from build123d import *

# Parameters (mm, degrees)
F1_DEPTH  = 15.875
F2_R      = 38.1
F3_DEPTH  = 31.751
F5_DEPTH  = 25.4
F6_R      = 12.7
F7_DEPTH  = 152.401
F9_DEPTH  = 25.4
F10_R     = 12.7
F11_DEPTH = 152.401
F14_DEPTH = 152.401


with BuildPart() as f1:
    # F0 (on Front) → F1 (new body, symmetric)
    with BuildSketch(Plane.XZ):
        with BuildLine():
            Line((88.9, 76.2), (0, 76.2))
            ThreePointArc((0, 76.2), (-76.2, 0), (0, -76.2))
            Line((0, -76.2), (88.9, -76.2))
            Line((88.9, -76.2), (88.9, 76.2))
        make_face()
    extrude(amount=F1_DEPTH, both=True)

    # F2 (on face) → F3 (cut, through all)
    with BuildSketch(Plane.XZ.offset(15.875)):
        Circle(F2_R)
    extrude(amount=-F3_DEPTH, mode=Mode.SUBTRACT)

    # F4 (on face) → F5 (join)
    with BuildSketch(Plane.XY.offset(76.2)):
        with BuildLine():
            ThreePointArc((114.3, -15.875), (142.540126, -23.966517), (159.527869, 0))
            ThreePointArc((159.527869, 0), (142.540126, 23.966517), (114.3, 15.875))
            ThreePointArc((114.3, 15.875), (108.727869, 0), (114.3, -15.875))
        make_face()
        with BuildLine():
            Line((114.3, 15.875), (88.9, 15.875))
            Line((88.9, 15.875), (88.9, -15.875))
            Line((88.9, -15.875), (114.3, -15.875))
            ThreePointArc((114.3, -15.875), (108.727869, 0), (114.3, 15.875))
        make_face()
    extrude(amount=-F5_DEPTH)

    # F6 (on face) → F7 (cut, through all)
    with BuildSketch(Plane(origin=(0, 0, -76.2), x_dir=(1, 0, 0), z_dir=(0, 0, -1))):
        with Locations((134.127869, 0)):
            Circle(F6_R)
    extrude(amount=-F7_DEPTH, mode=Mode.SUBTRACT)

    # F8 (on face) → F9 (join)
    with BuildSketch(Plane(origin=(0, 0, -76.2), x_dir=(1, 0, 0), z_dir=(0, 0, -1))):
        with BuildLine():
            Line((114.3, 15.875), (88.9, 15.875))
            Line((88.9, 15.875), (88.9, -15.875))
            Line((88.9, -15.875), (114.3, -15.875))
            ThreePointArc((114.3, -15.875), (108.727869, 0), (114.3, 15.875))
        make_face()
        with BuildLine():
            ThreePointArc((159.527869, 0), (142.540126, 23.966517), (114.3, 15.875))
            ThreePointArc((114.3, 15.875), (108.727869, 0), (114.3, -15.875))
            ThreePointArc((114.3, -15.875), (142.540126, -23.966517), (159.527869, 0))
        make_face()
    extrude(amount=-F9_DEPTH)

    # F10 (on face) → F11 (cut, through all)
    with BuildSketch(Plane.XY.offset(76.2)):
        with Locations((134.127869, 0)):
            Circle(F10_R)
    extrude(amount=-F11_DEPTH, mode=Mode.SUBTRACT)

    # F13 (on face) → F14 (cut, through all)
    with BuildSketch(Plane.XY.offset(76.2)):
        with BuildLine():
            Line((70.627869, 6.35), (19.827869, 6.35))
            ThreePointArc((19.827869, 6.35), (13.477869, 0), (19.827869, -6.35))
            Line((19.827869, -6.35), (70.627869, -6.35))
            ThreePointArc((70.627869, -6.35), (76.977869, 0), (70.627869, 6.35))
        make_face()
    extrude(amount=-F14_DEPTH, mode=Mode.SUBTRACT)


solid = f1.part
Geometry: final body of the model. Coordinates: model frame, mm. A direction names the side the tool comes from. Coordinates: 2 decimals unless noted, no trailing zeros. Loops run counter-clockwise (first coordinate to the right, second up) from the corner with the lowest first, then second, coordinate; pieces in that order, holes last. Notation, with made-up numbers: (7.25, 19.5) - (22.25, 19.5) arc R25 ccw to (22.25, 46.5) - close; hole circle Ø10 at (2, 55.5). An arc over 180 degrees is marked (long way). One line per question, with ' | ' between items. Start each with the question number.
(1) Ray query, L1, parallel to Y at x = 37, z = 65 (3 decimals); L2, parallel to Z at x = 149, y = 0; L3, parallel to X at y = -6.5, z = -4. Return the intervals inside material, ascending. Write a range as from..to.
(2) Cut plane D-D on x = 25. Output: boundary loops of the cut face in (y, z) (3 decimals).
(3) Cut plane C-C on x = 135.5. Output: boundary loops of the cut face in (y, z), and give its area (3 significant figures).
(4) Reachability of faces 1 (the flat face through (42, -15.875, -1)), 2 (the flat face through (96, 0, 76.2)), 3 (the flat face through (39, 15.875, -1)), 4 (the flat face through (116, 0, 50.8)), 5 (the cylindrical face through (13.48, 0.14, 54.67)) from +Z, -Z, +X, -X, +Y, -Y: full face, straight path, thin tool, end or side. Return the list, or none.
(5) Cut plane A-A on z = 0. Output: boundary loops of the cut face in (x, y) (3 decimals), and give its area (3 significant figures).
(6) Cut plane B-B on x = 59. Output: boundary loops of the cut face in (y, z) (3 decimals), and give its area (3 significant figures).
(7) First-contact query: pin 1 (15 mm diameter, centred on x = 134.13, y = 0, fed in from +Z); pin 2 (16 mm diameter, centred on y = 1, z = -17.5, fed in from +X); pin 3 (4 mm diameter, centred on x = 48, z = 27.5, fed in from +Y) (3 decimals); pin 4 (2 mm diameter, centred on x = -50.5, z = 56, fed in from -Y) (3 decimals). Flat tips, straight axial feed; report the tip coordinate or a pass-through.
(8) Draft query along Z for faces 6 (the flat face through (116, 0, -50.8)), 7 (the cylindrical face through (-76.18, -0.22, 1.68)), 8 (the cylindrical face through (121.44, -0.56, 63.32)). Return one class per face: +Z half, -Z half, draft (parallel to the pull), parting line (faces both ways), or undercut.
Here are the results:
1) L1: -15.875..-6.35, 6.35..15.875 | L2: -76.2..-50.8, 50.8..76.2 | L3: -76.09..-37.89, 37.89..88.9
2) outline: (-15.875, -76.2) - (-6.35, -76.2) - (-6.35, -28.751) - (-15.875, -28.751) - close; (-15.875, 28.751) - (-6.35, 28.751) - (-6.35, 76.2) - (-15.875, 76.2) - close; (6.35, -76.2) - (15.875, -76.2) - (15.875, -28.751) - (6.35, -28.751) - close; (6.35, 28.751) - (15.875, 28.751) - (15.875, 76.2) - (6.35, 76.2) - close
3) outline: (-25.36, -76.2) - (-12.63, -76.2) - (-12.63, -50.8) - (-25.36, -50.8) - close; (-25.36, 50.8) - (-12.63, 50.8) - (-12.63, 76.2) - (-25.36, 76.2) - close; (12.63, -76.2) - (25.36, -76.2) - (25.36, -50.8) - (12.63, -50.8) - close; (12.63, 50.8) - (25.36, 50.8) - (25.36, 76.2) - (12.63, 76.2) - close | area: 1,290 mm²
4) face 1: +Z, -Z, -X, -Y | face 2: +Z, +X, -X, +Y, -Y | face 3: +Z, -Z, -X, +Y | face 4: +X, +Y, -Y | face 5: +Z, -Z
5) outline: (-76.2, -15.875) - (-38.1, -15.875) - (-38.1, 15.875) - (-76.2, 15.875) - close; (38.1, -15.875) - (88.9, -15.875) - (88.9, 15.875) - (38.1, 15.875) - (38.1, 6.35) - (70.628, 6.35) arc R6.35 cw to (70.628, -6.35) - (38.1, -6.35) - close | area: 2,350 mm²
6) outline: (-15.875, -76.2) - (-6.35, -76.2) - (-6.35, 76.2) - (-15.875, 76.2) - close; (6.35, -76.2) - (15.875, -76.2) - (15.875, 76.2) - (6.35, 76.2) - close | area: 2,900 mm²
7) pin 1: through | pin 2: x = 88.9 | pin 3: y = 15.875 | pin 4: y = -15.875
8) face 6: undercut | face 7: parting line | face 8: draft
